Drawing for the job (mm, zero at the part's lowest x, y, z). A direction names the side the tool comes from. Round coordinates to 2 decimals unless told otherwise and drop trailing zeros. Write each loop counter-clockwise with the first axis right and the second up, starting at its lowest first coordinate (ties: lowest second). Pieces come first, ordered by that corner, then holes. Notation, with made-up numbers: (15.25, -13) - (28.25, -13) arc R18 cw to (28.25, 3) - close; hole circle Ø5 at (61.5, 23.25). An arc over 180 degrees is marked (long way). Answer in a Markdown table with one row per item.
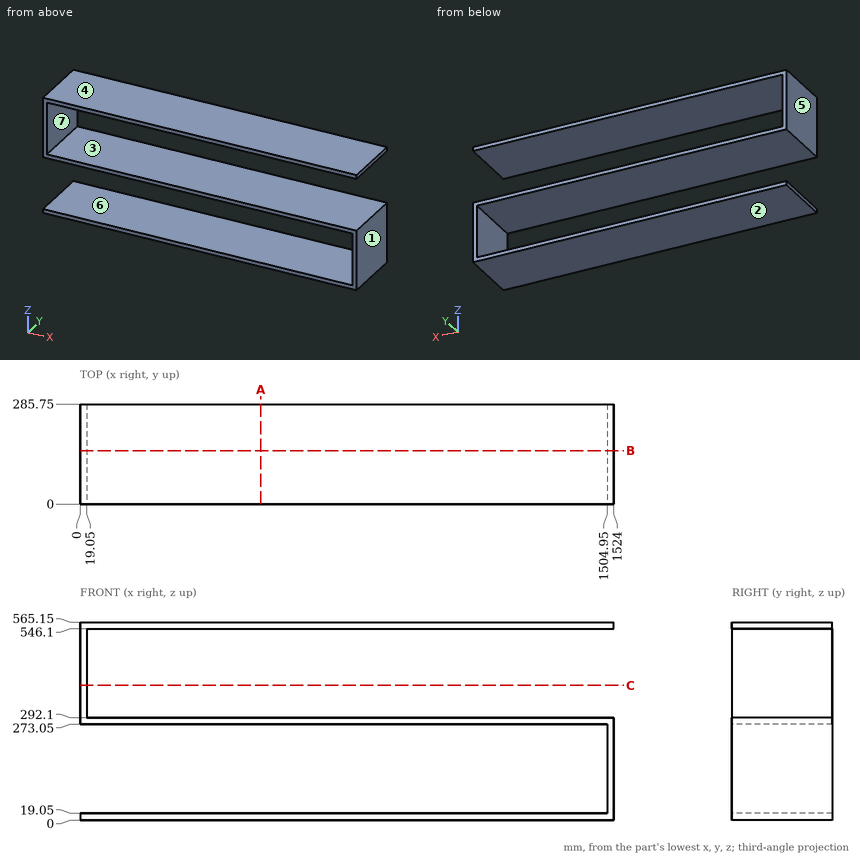
Q1. Saw through at A-A on x = 516.5. List the corners of the cut face in (y, z), then the cut area to 3 significant figures.
Computed:
| item | result |
|---|---|
| outline | (0, 0) - (285.75, 0) - (285.75, 19.05) - (0, 19.05) - close; (0, 273.05) - (285.75, 273.05) - (285.75, 292.1) - (0, 292.1) - close; (0, 546.1) - (285.75, 546.1) - (285.75, 565.15) - (0, 565.15) - close |
| area | 16,300 mm2 |
Q2. Saw through at C-C on z = 384.5. List the corners of the cut face in (x, y), then the cut area to 3 significant figures.
Computed:
| item | result |
|---|---|
| outline | (0, 0) - (19.05, 0) - (19.05, 285.75) - (0, 285.75) - close |
| area | 5,440 mm2 |
Q3. Drill centre lines: line 1 (Z direction, x = 1121, y = 183); line 2 (X direction, y = 64.5, z = 397.5); line 3 (X direction, y = 69, z = 234.5). Where is each one in solid material? Low to high.
Computed:
| item | result |
|---|---|
| line 1 | z = 0 to 19.05, 273.05 to 292.1, 546.1 to 565.15 |
| line 2 | x = 0 to 19.05 |
| line 3 | x = 1504.95 to 1524 |
Q4. Saw through at B-B on y = 153. List the corners of the cut face in (x, z).
Computed:
| item | result |
|---|---|
| outline | (0, 0) - (1524, 0) - (1524, 292.1) - (19.05, 292.1) - (19.05, 546.1) - (1524, 546.1) - (1524, 565.15) - (0, 565.15) - (0, 273.05) - (1504.95, 273.05) - (1504.95, 19.05) - (0, 19.05) - close |
Q5. Flat gauge pins, fed straight in: pin 1 (2 mm diameter, centred on y = 228.5, z = 255.5, fed in from -X); pin 2 (1 mm diameter, centred on y = 191, z = 408.5, fed in from +X). Where does each tip first touch, or does it go through?
Computed:
| item | result |
|---|---|
| pin 1 | stops at x = 1504.95 |
| pin 2 | stops at x = 19.05 |
Q6. Pull direction Z, two halves, no side cores. Call the marked faces 1, 2, 3 and 4: released by +Z, released by -Z, zero draft, split by the parting line, or undercut.
Computed:
| item | result |
|---|---|
| face 1 | zero draft |
| face 2 | released by -Z |
| face 3 | undercut |
| face 4 | released by +Z |
Q7. 3-axis set-ups, long thin cutter, end or side, ignore diameter. For the marked faces 5, 6 and 7: which of +Z, -Z, +X, -X, +Y, -Y reach the whole face in a straight line?
Computed:
| item | result |
|---|---|
| face 5 | +Z, -Z, -X, +Y, -Y |
| face 6 | -X, +Y, -Y |
| face 7 | +X, +Y, -Y |
